from build123d import *

# Parameters (mm, degrees)
BOX272_W        = 97
BOX272_H        = 22
BOX272_DEPTH    = 45
FILLET031_R     = 10.9
BOX274_W        = 8
BOX274_H        = 8
BOX274_DEPTH    = 3
CHAMFER049_SIZE = 7.9
BOX266_W        = 3
BOX266_H        = 5
BOX266_DEPTH    = 50
BOX265_W        = 3
BOX265_H        = 42
BOX265_DEPTH    = 10
BOX264_W        = 3
BOX264_H        = 42
BOX264_DEPTH    = 10
BOX275_W        = 8
BOX275_H        = 8
BOX275_DEPTH    = 3
CHAMFER050_SIZE = 7.9


with BuildPart() as battery_pack001:
    # Box272 → Box272 (new body)
    with BuildSketch(Plane.XY):
        with Locations((48.5, 11)):
            Rectangle(BOX272_W, BOX272_H)
    extrude(amount=BOX272_DEPTH)

    # Fillet031
    fillet031_edges = [battery_pack001.edges().sort_by_distance(p)[0] for p in [
        (48.5, 0, 0),
        (48.5, 0, 45),
        (48.5, 22, 0),
        (48.5, 22, 45),
    ]]
    fillet(fillet031_edges, radius=FILLET031_R)


with BuildPart() as battery_pack001_1:
    # Fillet031 placement: moved
    add(battery_pack001.part.moved(Location((0, 0, 2.5))))


with BuildPart() as chamfer049:
    # Box274 → Box274 (new body)
    with BuildSketch(Plane(origin=(3, 32, 0), x_dir=(1, 0, 0), z_dir=(0, 0, 1))):
        with Locations((4, 4)):
            Rectangle(BOX274_W, BOX274_H)
    extrude(amount=BOX274_DEPTH)

    # Chamfer049
    chamfer049_edges = [chamfer049.edges().sort_by_distance(p)[0] for p in [
        (11, 32, 1.5),
    ]]
    chamfer(chamfer049_edges, length=CHAMFER049_SIZE)


with BuildPart() as chamfer049_1:
    # Chamfer049 placement: moved
    add(chamfer049.part.moved(Location((0, 2, 47))))


with BuildPart() as cube238:
    # Box266 → Box266 (new body)
    with BuildSketch(Plane(origin=(0, 37, 0), x_dir=(1, 0, 0), z_dir=(0, 0, 1))):
        with Locations((1.5, 2.5)):
            Rectangle(BOX266_W, BOX266_H)
    extrude(amount=BOX266_DEPTH)


with BuildPart() as cube237:
    # Box265 → Box265 (new body)
    with BuildSketch(Plane.XY.offset(40)):
        with Locations((1.5, 21)):
            Rectangle(BOX265_W, BOX265_H)
    extrude(amount=BOX265_DEPTH)


with BuildPart() as cube236:
    # Box264 → Box264 (new body)
    with BuildSketch(Plane.XY):
        with Locations((1.5, 21)):
            Rectangle(BOX264_W, BOX264_H)
    extrude(amount=BOX264_DEPTH)


with BuildPart() as cut:
    # Box275 → Box275 (new body)
    with BuildSketch(Plane(origin=(3, 32, 0), x_dir=(1, 0, 0), z_dir=(0, 0, 1))):
        with Locations((4, 4)):
            Rectangle(BOX275_W, BOX275_H)
    extrude(amount=BOX275_DEPTH)

    # Chamfer050
    chamfer050_edges = [cut.edges().sort_by_distance(p)[0] for p in [
        (11, 32, 1.5),
    ]]
    chamfer(chamfer050_edges, length=CHAMFER050_SIZE)


with BuildPart() as cut_1:
    # Chamfer050 placement: moved
    add(cut.part.moved(Location((0, 2, 0))))

    # Fusion073: union Chamfer049, Cube238, Cube237, Cube236
    add(chamfer049_1.part)
    add(cube238.part)
    add(cube237.part)
    add(cube236.part)

    # Cut: cut Battery pack001
    add(battery_pack001_1.part, mode=Mode.SUBTRACT)


solid = cut_1.part
The model under review builds one solid part; all positions refer to its coordinate system, in mm. A direction names the side the tool comes from. Coordinates: 2 decimals unless noted, no trailing zeros. Write each loop counter-clockwise with the first axis right and the second up, starting at its lowest first coordinate (ties: lowest second). Pieces come first, ordered by that corner, then holes. Notation, with made-up numbers: (-25, -31.5) -> (12, -31.5) arc R28 cw to (12, 0.5) -> close; hole circle Ø7 at (25.5, 78.25). An arc over 180 degrees is marked (long way). Answer in a Markdown table with one row per item.
1. We need section C-C, the plane x = 1.25. State the section outline as (y, z) points.
Answers below:
| item | result |
|---|---|
| outline | (0, 0) -> (42, 0) -> (42, 50) -> (0, 50) -> (0, 40) -> (0.54, 40) arc R10.9 cw to (10.9, 47.5) -> (11.1, 47.5) arc R10.9 cw to (21.46, 40) -> (37, 40) -> (37, 10) -> (21.46, 10) arc R10.9 cw to (11.1, 2.5) -> (10.9, 2.5) arc R10.9 cw to (0.54, 10) -> (0, 10) -> close |
2. For faces 1 (the flat face through (2, 42, 19)), 2 (the flat face through (1, 29, 40)), 3 (the cylindrical face through (1.52, 4.43, 4.63)), 4 (the flat face through (6, 39, 3)), list the 3-axis set-ups (+Z, -Z, +X, -X, +Y, -Y) from which the entire face can be reached by the end or side of a thin tool; tool diameter is ignored.
Answers below:
| item | result |
|---|---|
| face 1 | +Z, -Z, +X, -X, +Y |
| face 2 | +X, -X, -Y |
| face 3 | +X, -X |
| face 4 | +X, +Y, -Y |
3. Wall thickness on probe 1 along Z at (x, y) = (2, 32); probe 2 along Y at (x, z) = (2.75, 21); probe 3 along X at (y, z) = (2, 46): over which ranges is each line inside the solid? List them lowest first. Write a range as [from, to].
Answers below:
| item | result |
|---|---|
| probe 1 | z = [0, 10], [40, 50] |
| probe 2 | y = [37, 42] |
| probe 3 | x = [0, 3] |
4. We need section A-A, the plane x = 7.25. State the section outline as (y, z) points, and give its area (3 significant figures).
Answers below:
| item | result |
|---|---|
| outline | (38.15, 0) -> (42, 0) -> (42, 3) -> (38.15, 3) -> close; (38.15, 47) -> (42, 47) -> (42, 50) -> (38.15, 50) -> close |
| area | 23.1 mm^2 |
5. We need section D-D, the plane z = 38. State the section outline as (x, y) points, and give its area (3 significant figures).
Answers below:
| item | result |
|---|---|
| outline | (0, 37) -> (3, 37) -> (3, 42) -> (0, 42) -> close |
| area | 15.0 mm^2 |
6. We need section B-B, the plane y = 25.5. State the section outline as (x, z) points.
Answers below:
| item | result |
|---|---|
| outline | (0, 0) -> (3, 0) -> (3, 10) -> (0, 10) -> close; (0, 40) -> (3, 40) -> (3, 50) -> (0, 50) -> close |
7. Clearance check with flat-ended pins moving along their axes: pin 1 Ø10 at (y, z) = (15.5, 39.5) entering from -X; pin 2 Ø1 at (y, z) = (29.5, 6.5) entering from +X; pin 3 Ø1.5 at (x, z) = (2, 27.5) entering from -Y. State where each tip first meets the part, or that it passes through.
Answers below:
| item | result |
|---|---|
| pin 1 | passes through |
| pin 2 | stops at x = 3 |
| pin 3 | stops at y = 37 |
8. Draft analysis for pull direction Z (two halves, no side actions). For faces 5 (the cylindrical face through (1.52, 17.57, 4.63)), 6 (the flat face through (7.1, 38, 48.5)), 7 (the flat face through (2, 26, 50)), state which applies: +Z half, -Z half, draft (parallel to the pull), parting line (faces both ways), or undercut.
Answers below:
| item | result |
|---|---|
| face 5 | undercut |
| face 6 | draft |
| face 7 | +Z half |
